Verification items for this drawing (mm, ordinates from the low corner). A direction names the side the tool comes from. Coordinates: 2 decimals unless noted, no trailing zeros. Write each loop counter-clockwise with the first axis right and the second up, starting at its lowest first coordinate (ties: lowest second). Pieces come first, ordered by that corner, then holes. Notation, with made-up numbers: M 57,-14 L 85,-14 A34 cw 85,25 Z; hole C -8.75,64 d4. An arc over 180 degrees is marked long. Put each result on its own line as item: value. Start each with the question number.
1) Scan lines: line 1 along Y through (x, z) = (16, 2.6); line 2 along Y through (x, z) = (16, 15.25); line 3 along X through (y, z) = (28.5, 3). Record each from-to range of solid material in increasing order.
2) Set-up check for the marked faces 4 and 5: record each of +Z, -Z, +X, -X, +Y, -Y from which the full face is reachable in a straight line by a thin tool's end or side.
3) Cross-section at D-D on z = 13.75. Record the cut outline in (x, y), plus the area to 3 significant figures.
4) Gauge pin test, flat ends, axial feed: pin 1 (1 mm diameter, centred on x = 26.5, z = 3.5, fed in from -Y); pin 2 (2 mm diameter, centred on y = 9, z = 8.5, fed in from +X); pin 3 (12 mm diameter, centred on y = 27, z = 16.5, fed in from -X); pin 4 (3 mm diameter, centred on x = 6.5, y = 20.5, fed in from +Z). Record the tip position at first contact, or that the pin passes through.
5) Cross-section at C-C on z = 2.5. Record the cut outline in (x, y).
6) Cross-section at A-A on x = 16. Record the cut outline in (y, z).
7) Mould release check, pull along Y, two halves, no side actions. Record for the marked faces 1, 2 and 3: released by +Y, released by -Y, zero draft, split by the parting line, or undercut.
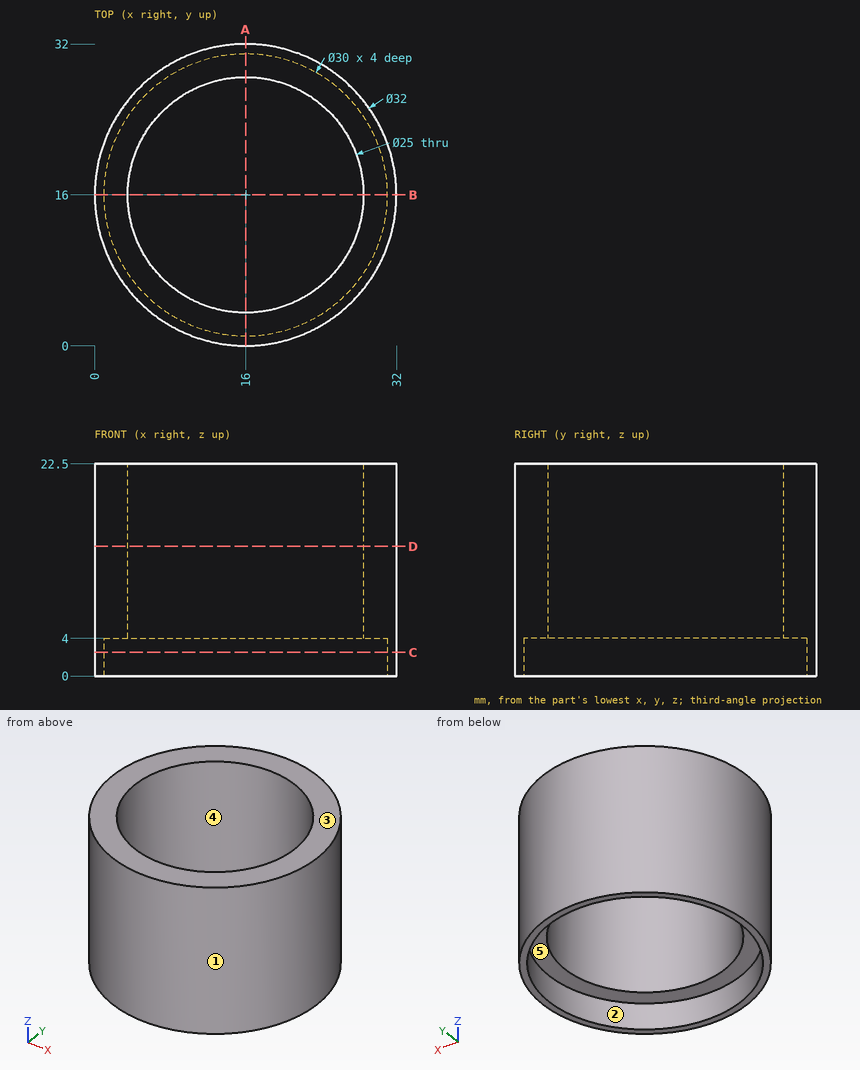
Answer key:
1. line 1: y = 0 to 1, 31 to 32
1. line 2: y = 0 to 3.5, 28.5 to 32
1. line 3: x = 6.01 to 7.71, 24.29 to 25.99
2. face 4: +Z, -Z
2. face 5: -Z
3. outline: C 16,16 d32; hole C 16,16 d25
3. area: 313 mm²
4. pin 1: stops at y = 3.51
4. pin 2: stops at x = 30.83
4. pin 3: stops at x = 0.8
4. pin 4: passes through
5. outline: C 16,16 d32; hole C 16,16 d30
6. outline: M 0,0 L 1,0 L 1,4 L 3.5,4 L 3.5,22.5 L 0,22.5 Z; M 28.5,4 L 31,4 L 31,0 L 32,0 L 32,22.5 L 28.5,22.5 Z
7. face 1: split by the parting line
7. face 2: undercut
7. face 3: zero draft
